CAD build for the part. Positions are in the model's coordinates, mm. Face numbers are marked on the shaded views. Give positions to 0.01 mm unless a question says otherwise; leave off trailing zeros. Loops run counter-clockwise (first coordinate to the right, second up) from the corner with the lowest first, then second, coordinate; pieces in that order, holes last. Notation, with made-up numbers: (76, 41.25) - (110, 41.25) arc R31 cw to (110, 78.25) - close; hole circle Ø8 at (-36, 29.5). An arc over 180 degrees is marked (long way). Return JSON: item names as keys, results as strings.
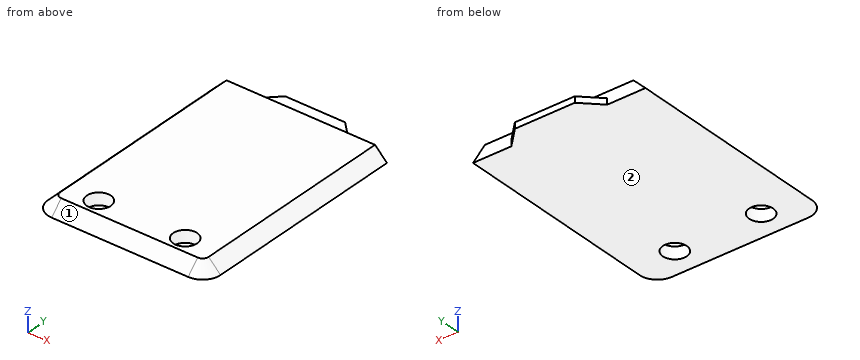
Autodesk Inventor part; units mm, degrees
ref_plane "YZ Plane" through (0, 0, 0) normal (1, 0, 0) x (0, 1, 0)
ref_plane "XZ Plane" through (0, 0, 0) normal (0, 1, 0) x (-1, 0, 0)
ref_plane "XY Plane" through (0, 0, 0) normal (0, 0, 1) x (1, 0, 0)
sketch "Skizze1" plane through (0, 0, 0) normal (0, 0, 1) x (1, 0, 0)
  line L0 (3.4, 37.6) -> (-3, 37.6)
  line L1 (-3, 37.6) -> (-3, 3)
  arc A0 (-3, 3) -> (0, 0) centre (0, 3) ccw
  line L2 (0, 0) -> (22.8, 0)
  arc A1 (22.8, 0) -> (25.8, 3) centre (22.8, 3) ccw
  line L3 (25.8, 3) -> (25.8, 37.6)
  line L4 (25.8, 37.6) -> (19.4, 37.6)
  line L5 (19.4, 37.6) -> (16.4, 40.6)
  line L6 (16.4, 40.6) -> (6.4, 40.6)
  line L7 (6.4, 40.6) -> (3.4, 37.6)
  line L8 (-1.8, 35.6) -> (24.6, 35.6)
  line L9 (24.6, 35.6) -> (24.6, 9.2)
  line L10 (24.6, 9.2) -> (-1.8, 9.2)
  line L11 (-1.8, 9.2) -> (-1.8, 35.6)
  line L12 (24.6, 35.6) -> (-1.8, 35.6)
  line L13 (-1.8, 35.6) -> (-1.8, 9.2)
  line L14 (-1.8, 9.2) -> (24.6, 9.2)
  line L15 (24.6, 9.2) -> (24.6, 35.6)
  line L16 (24.6, 35.6) -> (-1.8, 35.6)
  line L17 (-3, 37.6) -> (3.4, 37.6)
  line L18 (-3, 3) -> (-3, 37.6)
  arc A2 (-3, 3) -> (0, 0) centre (0, 3) ccw
  line L19 (22.8, 0) -> (0, 0)
  arc A3 (22.8, 0) -> (25.8, 3) centre (22.8, 3) ccw
  line L20 (25.8, 37.6) -> (25.8, 3)
  line L21 (19.4, 37.6) -> (25.8, 37.6)
  line L22 (19.4, 37.6) -> (16.4, 40.6)
  line L23 (16.4, 40.6) -> (6.4, 40.6)
  line L24 (6.4, 40.6) -> (3.4, 37.6)
  circle A4 centre (4.1926, 4.6) radius 2
  line L25 (11.4, 35.6) -> (11.4, 0)
  circle A5 centre (18.6074, 4.6) radius 2
  point P0 (-3, 37.6)
  point P1 (-3, 3)
  point P2 (0, 0)
extrude "Extrusion1" add sketch "Skizze1" along normal blind 2 contours L7 L6 L5 L4 L3 A1 L2 A0 L1 L0 | L8 L25 L10 L11 | L8 L9 L10 L25
chamfer "Fase1" distance 2 angle 45 5 edges at (25.8, 20.3, 2) (24.9213, 0.8787, 2) (11.4, 0, 2) (-2.1213, 0.8787, 2) (-3, 20.3, 2)
sketch "Skizze2" plane through (0, 0, 2) normal (0, 0, 1) x (1, 0, 0)
  line L0 (-1, 3) -> (-1, 37.6)
  arc A0 (-1, 3) -> (0, 2) centre (0, 3) ccw
  line L1 (22.8, 2) -> (0, 2)
  arc A1 (22.8, 2) -> (23.8, 3) centre (22.8, 3) ccw
  line L2 (23.8, 37.6) -> (23.8, 3)
  line L3 (23.8, 37.6) -> (19.4, 37.6)
  line L4 (19.4, 37.6) -> (16.4, 40.6)
  line L5 (16.4, 40.6) -> (6.4, 40.6)
  line L6 (6.4, 40.6) -> (3.4, 37.6)
  line L7 (3.4, 37.6) -> (-1, 37.6)
  line L8 (6.4, 40.6) -> (3.4, 37.6)
  line L9 (3.4, 37.6) -> (19.4, 37.6)
  point P0 (0, 0)
extrude "Extrusion2" cut sketch "Skizze2" against normal blind 1 contours L6 L5 L4 L9
properties part number "OBS-MainCase-A-004_GPS-Cover_v0.1.1"
1. Drop a flat-ended pin along its axis: P1, Ø2.5, axis at x = 11, y = 39, coming from the +Z side. Give the stop position or say it passes through.
Values follow:
{"P1": "stops at z = 1"}
2. Cut at A-A, the plane y = 4.6. Give the number of separate pieces and of enclosed holes in the cut face, plus the area to 3 significant figures.
Values follow:
{"separate pieces": "3", "enclosed holes": "0", "area": "37.6 mm²"}
3. Drill centre lines: probe 1 along X at (y, z) = (6, 0.8); probe 2 along Y at (x, z) = (5.5, 0.1); probe 3 along Z at (x, y) = (24.5, 17.5). Where is each one in solid material? Low to high.
Values follow:
{"probe 1": "x = -2.2 to 2.76, 5.62 to 17.18, 20.04 to 25", "probe 2": "y = 0.1 to 3.09, 6.11 to 39.7", "probe 3": "z = 0 to 1.3"}
4. Pull direction Z, two halves, no side cores. Call the marked faces 1 and 2: +Z half, -Z half, draft (parallel to the pull), parting line (faces both ways), or undercut.
Values follow:
{"face 1": "+Z half", "face 2": "-Z half"}
5. Cut at C-C, the plane z = 1.4. Write the cut outline in (x, y).
Values follow:
{"outline": "(-1.6, 3) arc R1.6 ccw to (0, 1.4) - (22.8, 1.4) arc R1.6 ccw to (24.4, 3) - (24.4, 37.6) - (-1.6, 37.6) - close; hole circle Ø4 at (4.19, 4.6); hole circle Ø4 at (18.61, 4.6)"}
